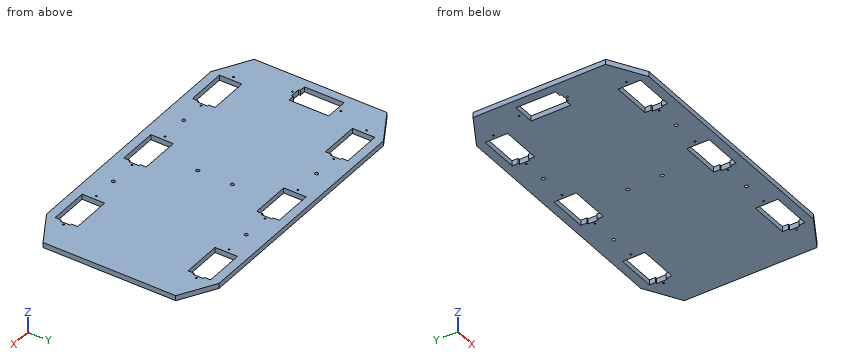
```python
from build123d import *

# Parameters (mm, degrees)
BOSS_EXTRUDE1_DEPTH = 3
CUT_EXTRUDE1_REACH  = 105
SKETCH2_R           = 0.5
SKETCH2_R_2         = 1
CUT_EXTRUDE2_REACH  = 105
SKETCH3_R           = 0.5
CUT_EXTRUDE3_REACH  = 105
SKETCH5_R           = 1


with BuildPart() as part:
    # Sketch1 → Boss-Extrude1 (new body)
    with BuildSketch(Plane.XY):
        Polygon((70, 50), (90, 38.452994616), (90, -38.452994616), (70, -50), (-70, -50), (-90, -38.452994616), (-90, 38.452994616), (-70, 50), align=None)
    extrude(amount=BOSS_EXTRUDE1_DEPTH)

    # Sketch2 → Cut-Extrude1 (cut, up to next)
    with BuildSketch(Plane.XY.offset(3), mode=Mode.PRIVATE) as cut_extrude1_sk1:
        with Locations((-72.5, 38.5)):
            Circle(SKETCH2_R)
    cut_extrude1_tool1 = extrude(cut_extrude1_sk1.sketch, amount=-CUT_EXTRUDE1_REACH, mode=Mode.PRIVATE) & part.part
    # Sketch2 → Cut-Extrude1 (cut, up to next)
    with BuildSketch(Plane.XY.offset(3), mode=Mode.PRIVATE) as cut_extrude1_sk2:
        with Locations((-44.5, 38.5)):
            Circle(SKETCH2_R)
    cut_extrude1_tool2 = extrude(cut_extrude1_sk2.sketch, amount=-CUT_EXTRUDE1_REACH, mode=Mode.PRIVATE) & part.part
    # Sketch2 → Cut-Extrude1 (cut, up to next)
    with BuildSketch(Plane.XY.offset(3), mode=Mode.PRIVATE) as cut_extrude1_sk3:
        with Locations((-14, 38.5)):
            Circle(SKETCH2_R)
    cut_extrude1_tool3 = extrude(cut_extrude1_sk3.sketch, amount=-CUT_EXTRUDE1_REACH, mode=Mode.PRIVATE) & part.part
    # Sketch2 → Cut-Extrude1 (cut, up to next)
    with BuildSketch(Plane.XY.offset(3), mode=Mode.PRIVATE) as cut_extrude1_sk4:
        with Locations((14, 38.5)):
            Circle(SKETCH2_R)
    cut_extrude1_tool4 = extrude(cut_extrude1_sk4.sketch, amount=-CUT_EXTRUDE1_REACH, mode=Mode.PRIVATE) & part.part
    # Sketch2 → Cut-Extrude1 (cut, up to next)
    with BuildSketch(Plane.XY.offset(3), mode=Mode.PRIVATE) as cut_extrude1_sk5:
        with Locations((44.5, 38.5)):
            Circle(SKETCH2_R)
    cut_extrude1_tool5 = extrude(cut_extrude1_sk5.sketch, amount=-CUT_EXTRUDE1_REACH, mode=Mode.PRIVATE) & part.part
    # Sketch2 → Cut-Extrude1 (cut, up to next)
    with BuildSketch(Plane.XY.offset(3), mode=Mode.PRIVATE) as cut_extrude1_sk6:
        with Locations((72.5, 38.5)):
            Circle(SKETCH2_R)
    cut_extrude1_tool6 = extrude(cut_extrude1_sk6.sketch, amount=-CUT_EXTRUDE1_REACH, mode=Mode.PRIVATE) & part.part
    # Sketch2 → Cut-Extrude1 (cut, up to next)
    with BuildSketch(Plane.XY.offset(3), mode=Mode.PRIVATE) as cut_extrude1_sk7:
        with Locations((72.5, -38.5)):
            Circle(SKETCH2_R)
    cut_extrude1_tool7 = extrude(cut_extrude1_sk7.sketch, amount=-CUT_EXTRUDE1_REACH, mode=Mode.PRIVATE) & part.part
    # Sketch2 → Cut-Extrude1 (cut, up to next)
    with BuildSketch(Plane.XY.offset(3), mode=Mode.PRIVATE) as cut_extrude1_sk8:
        with Locations((44.5, -38.5)):
            Circle(SKETCH2_R)
    cut_extrude1_tool8 = extrude(cut_extrude1_sk8.sketch, amount=-CUT_EXTRUDE1_REACH, mode=Mode.PRIVATE) & part.part
    # Sketch2 → Cut-Extrude1 (cut, up to next)
    with BuildSketch(Plane.XY.offset(3), mode=Mode.PRIVATE) as cut_extrude1_sk9:
        with Locations((14, -38.5)):
            Circle(SKETCH2_R)
    cut_extrude1_tool9 = extrude(cut_extrude1_sk9.sketch, amount=-CUT_EXTRUDE1_REACH, mode=Mode.PRIVATE) & part.part
    # Sketch2 → Cut-Extrude1 (cut, up to next)
    with BuildSketch(Plane.XY.offset(3), mode=Mode.PRIVATE) as cut_extrude1_sk10:
        with Locations((-14, -38.5)):
            Circle(SKETCH2_R)
    cut_extrude1_tool10 = extrude(cut_extrude1_sk10.sketch, amount=-CUT_EXTRUDE1_REACH, mode=Mode.PRIVATE) & part.part
    # Sketch2 → Cut-Extrude1 (cut, up to next)
    with BuildSketch(Plane.XY.offset(3), mode=Mode.PRIVATE) as cut_extrude1_sk11:
        with Locations((-44.5, -38.5)):
            Circle(SKETCH2_R)
    cut_extrude1_tool11 = extrude(cut_extrude1_sk11.sketch, amount=-CUT_EXTRUDE1_REACH, mode=Mode.PRIVATE) & part.part
    # Sketch2 → Cut-Extrude1 (cut, up to next)
    with BuildSketch(Plane.XY.offset(3), mode=Mode.PRIVATE) as cut_extrude1_sk12:
        with Locations((-72.5, -38.5)):
            Circle(SKETCH2_R)
    cut_extrude1_tool12 = extrude(cut_extrude1_sk12.sketch, amount=-CUT_EXTRUDE1_REACH, mode=Mode.PRIVATE) & part.part
    # Sketch2 → Cut-Extrude1 (cut, up to next)
    with BuildSketch(Plane.XY.offset(3), mode=Mode.PRIVATE) as cut_extrude1_sk13:
        with Locations((0, 10)):
            Circle(SKETCH2_R_2)
    cut_extrude1_tool13 = extrude(cut_extrude1_sk13.sketch, amount=-CUT_EXTRUDE1_REACH, mode=Mode.PRIVATE) & part.part
    # Sketch2 → Cut-Extrude1 (cut, up to next)
    with BuildSketch(Plane.XY.offset(3), mode=Mode.PRIVATE) as cut_extrude1_sk14:
        with Locations((0, -10)):
            Circle(SKETCH2_R_2)
    cut_extrude1_tool14 = extrude(cut_extrude1_sk14.sketch, amount=-CUT_EXTRUDE1_REACH, mode=Mode.PRIVATE) & part.part
    # Sketch2 → Cut-Extrude1 (cut, up to next)
    with BuildSketch(Plane.XY.offset(3), mode=Mode.PRIVATE) as cut_extrude1_sk15:
        Polygon((-11.5, 45), (11.5, 45), (11.5, 41.5), (12.5, 41.5), (12.5, 35.5), (11.5, 35.5), (11.5, 32), (-11.5, 32), align=None)
    cut_extrude1_tool15 = extrude(cut_extrude1_sk15.sketch, amount=-CUT_EXTRUDE1_REACH, mode=Mode.PRIVATE) & part.part
    # Sketch2 → Cut-Extrude1 (cut, up to next)
    with BuildSketch(Plane.XY.offset(3), mode=Mode.PRIVATE) as cut_extrude1_sk16:
        Polygon((-11.5, -32), (11.5, -32), (11.5, -35.5), (12.5, -35.5), (12.5, -41.5), (11.5, -41.5), (11.5, -45), (-11.5, -45), align=None)
    cut_extrude1_tool16 = extrude(cut_extrude1_sk16.sketch, amount=-CUT_EXTRUDE1_REACH, mode=Mode.PRIVATE) & part.part
    # Sketch2 → Cut-Extrude1 (cut, up to next)
    with BuildSketch(Plane.XY.offset(3), mode=Mode.PRIVATE) as cut_extrude1_sk17:
        Polygon((-70, 45), (-47, 45), (-47, 41.5), (-46, 41.5), (-46, 35.5), (-47, 35.5), (-47, 32), (-70, 32), align=None)
    cut_extrude1_tool17 = extrude(cut_extrude1_sk17.sketch, amount=-CUT_EXTRUDE1_REACH, mode=Mode.PRIVATE) & part.part
    # Sketch2 → Cut-Extrude1 (cut, up to next)
    with BuildSketch(Plane.XY.offset(3), mode=Mode.PRIVATE) as cut_extrude1_sk18:
        Polygon((-70, -32), (-47, -32), (-47, -35.5), (-46, -35.5), (-46, -41.5), (-47, -41.5), (-47, -45), (-70, -45), align=None)
    cut_extrude1_tool18 = extrude(cut_extrude1_sk18.sketch, amount=-CUT_EXTRUDE1_REACH, mode=Mode.PRIVATE) & part.part
    # Sketch2 → Cut-Extrude1 (cut, up to next)
    with BuildSketch(Plane.XY.offset(3), mode=Mode.PRIVATE) as cut_extrude1_sk19:
        Polygon((70, -32), (47, -32), (47, -45), (70, -45), (70, -41.5), (71, -41.5), (71, -35.5), (70, -35.5), align=None)
    cut_extrude1_tool19 = extrude(cut_extrude1_sk19.sketch, amount=-CUT_EXTRUDE1_REACH, mode=Mode.PRIVATE) & part.part
    # Sketch2 → Cut-Extrude1 (cut, up to next)
    with BuildSketch(Plane.XY.offset(3), mode=Mode.PRIVATE) as cut_extrude1_sk20:
        Polygon((70, 45), (47, 45), (47, 32), (70, 32), (70, 35.5), (71, 35.5), (71, 41.5), (70, 41.5), align=None)
    cut_extrude1_tool20 = extrude(cut_extrude1_sk20.sketch, amount=-CUT_EXTRUDE1_REACH, mode=Mode.PRIVATE) & part.part
    add(cut_extrude1_tool1.solids().sort_by_distance((-72.5, 38.5, 3))[0], mode=Mode.SUBTRACT)
    add(cut_extrude1_tool2.solids().sort_by_distance((-44.5, 38.5, 3))[0], mode=Mode.SUBTRACT)
    add(cut_extrude1_tool3.solids().sort_by_distance((-14, 38.5, 3))[0], mode=Mode.SUBTRACT)
    add(cut_extrude1_tool4.solids().sort_by_distance((14, 38.5, 3))[0], mode=Mode.SUBTRACT)
    add(cut_extrude1_tool5.solids().sort_by_distance((44.5, 38.5, 3))[0], mode=Mode.SUBTRACT)
    add(cut_extrude1_tool6.solids().sort_by_distance((72.5, 38.5, 3))[0], mode=Mode.SUBTRACT)
    add(cut_extrude1_tool7.solids().sort_by_distance((72.5, -38.5, 3))[0], mode=Mode.SUBTRACT)
    add(cut_extrude1_tool8.solids().sort_by_distance((44.5, -38.5, 3))[0], mode=Mode.SUBTRACT)
    add(cut_extrude1_tool9.solids().sort_by_distance((14, -38.5, 3))[0], mode=Mode.SUBTRACT)
    add(cut_extrude1_tool10.solids().sort_by_distance((-14, -38.5, 3))[0], mode=Mode.SUBTRACT)
    add(cut_extrude1_tool11.solids().sort_by_distance((-44.5, -38.5, 3))[0], mode=Mode.SUBTRACT)
    add(cut_extrude1_tool12.solids().sort_by_distance((-72.5, -38.5, 3))[0], mode=Mode.SUBTRACT)
    add(cut_extrude1_tool13.solids().sort_by_distance((0, 10, 3))[0], mode=Mode.SUBTRACT)
    add(cut_extrude1_tool14.solids().sort_by_distance((0, -10, 3))[0], mode=Mode.SUBTRACT)
    add(cut_extrude1_tool15.solids().sort_by_distance((0.236066, 38.5, 3))[0], mode=Mode.SUBTRACT)
    add(cut_extrude1_tool16.solids().sort_by_distance((0.236066, -38.5, 3))[0], mode=Mode.SUBTRACT)
    add(cut_extrude1_tool17.solids().sort_by_distance((-58.263934, 38.5, 3))[0], mode=Mode.SUBTRACT)
    add(cut_extrude1_tool18.solids().sort_by_distance((-58.263934, -38.5, 3))[0], mode=Mode.SUBTRACT)
    add(cut_extrude1_tool19.solids().sort_by_distance((58.736066, -38.5, 3))[0], mode=Mode.SUBTRACT)
    add(cut_extrude1_tool20.solids().sort_by_distance((58.736066, 38.5, 3))[0], mode=Mode.SUBTRACT)

    # Sketch3 → Cut-Extrude2 (cut, up to next)
    with BuildSketch(Plane.XY.offset(3), mode=Mode.PRIVATE) as cut_extrude2_sk1:
        with Locations((-78.5, 19.5)):
            Circle(SKETCH3_R)
    cut_extrude2_tool1 = extrude(cut_extrude2_sk1.sketch, amount=-CUT_EXTRUDE2_REACH, mode=Mode.PRIVATE) & part.part
    # Sketch3 → Cut-Extrude2 (cut, up to next)
    with BuildSketch(Plane.XY.offset(3), mode=Mode.PRIVATE) as cut_extrude2_sk2:
        with Locations((-78.5, -8.5)):
            Circle(SKETCH3_R)
    cut_extrude2_tool2 = extrude(cut_extrude2_sk2.sketch, amount=-CUT_EXTRUDE2_REACH, mode=Mode.PRIVATE) & part.part
    # Sketch3 → Cut-Extrude2 (cut, up to next)
    with BuildSketch(Plane.XY.offset(3), mode=Mode.PRIVATE) as cut_extrude2_sk3:
        Polygon((-85, 17), (-72, 17), (-72, -6), (-75.5, -6), (-75.5, -7), (-81.5, -7), (-81.5, -6), (-85, -6), align=None)
    cut_extrude2_tool3 = extrude(cut_extrude2_sk3.sketch, amount=-CUT_EXTRUDE2_REACH, mode=Mode.PRIVATE) & part.part
    add(cut_extrude2_tool1.solids().sort_by_distance((-78.5, 19.5, 3))[0], mode=Mode.SUBTRACT)
    add(cut_extrude2_tool2.solids().sort_by_distance((-78.5, -8.5, 3))[0], mode=Mode.SUBTRACT)
    add(cut_extrude2_tool3.solids().sort_by_distance((-78.5, 5.263934, 3))[0], mode=Mode.SUBTRACT)

    # Sketch5 → Cut-Extrude3 (cut, up to next)
    with BuildSketch(Plane(origin=(0, 0, 0), x_dir=(-1, 0, 0), z_dir=(0, 0, -1)), mode=Mode.PRIVATE) as cut_extrude3_sk1:
        with Locations((30, 38.5)):
            Circle(SKETCH5_R)
    cut_extrude3_tool1 = extrude(cut_extrude3_sk1.sketch, amount=-CUT_EXTRUDE3_REACH, mode=Mode.PRIVATE) & part.part
    # Sketch5 → Cut-Extrude3 (cut, up to next)
    with BuildSketch(Plane(origin=(0, 0, 0), x_dir=(-1, 0, 0), z_dir=(0, 0, -1)), mode=Mode.PRIVATE) as cut_extrude3_sk2:
        with Locations((-30, 38.5)):
            Circle(SKETCH5_R)
    cut_extrude3_tool2 = extrude(cut_extrude3_sk2.sketch, amount=-CUT_EXTRUDE3_REACH, mode=Mode.PRIVATE) & part.part
    # Sketch5 → Cut-Extrude3 (cut, up to next)
    with BuildSketch(Plane(origin=(0, 0, 0), x_dir=(-1, 0, 0), z_dir=(0, 0, -1)), mode=Mode.PRIVATE) as cut_extrude3_sk3:
        with Locations((30, -38.5)):
            Circle(SKETCH5_R)
    cut_extrude3_tool3 = extrude(cut_extrude3_sk3.sketch, amount=-CUT_EXTRUDE3_REACH, mode=Mode.PRIVATE) & part.part
    # Sketch5 → Cut-Extrude3 (cut, up to next)
    with BuildSketch(Plane(origin=(0, 0, 0), x_dir=(-1, 0, 0), z_dir=(0, 0, -1)), mode=Mode.PRIVATE) as cut_extrude3_sk4:
        with Locations((-30, -38.5)):
            Circle(SKETCH5_R)
    cut_extrude3_tool4 = extrude(cut_extrude3_sk4.sketch, amount=-CUT_EXTRUDE3_REACH, mode=Mode.PRIVATE) & part.part
    add(cut_extrude3_tool1.solids().sort_by_distance((-30, 38.5, 0))[0], mode=Mode.SUBTRACT)
    add(cut_extrude3_tool2.solids().sort_by_distance((30, 38.5, 0))[0], mode=Mode.SUBTRACT)
    add(cut_extrude3_tool3.solids().sort_by_distance((-30, -38.5, 0))[0], mode=Mode.SUBTRACT)
    add(cut_extrude3_tool4.solids().sort_by_distance((30, -38.5, 0))[0], mode=Mode.SUBTRACT)


solid = part.part
```
Check sheet for the modelled part. Datum: model origin and axes. Units: mm. Coordinates: 2 decimals unless noted, no trailing zeros. Order: outer loops, then holes, each group sorted by start corner. A loop starts at its lowest first (then second) coordinate and runs counter-clockwise, first axis right, second up. Notation, with made-up numbers: (70.5, -25) -> (80.5, -25) arc R18 ccw to (80.5, -3) -> close; hole circle Ø3 at (84, -1). An arc over 180 degrees is marked (long way). Write item = value, one per line. Start each with the question number.
1) Cross-section at A-A (x = 56.5). Enter the section's corners in (y, z), then the cut area to 3 significant figures.
2) Cross-section at B-B (y = 0). Enter the section's corners in (x, z), then the cut area to 3 significant figures.
3) Go/stop test with flat-tipped pins: P1, Ø0.9, axis at y = 43.5, z = 1, coming from the -X side; P2, Ø1.5, axis at y = 39.5, z = 1, coming from the +X side. Record where each tip stops, or that it passes through.
4) Material ranges on L1, parallel to Y at x = -14, z = 1.3; L2, parallel to Y at x = -56, z = 1.8; L3, parallel to X at y = 35, z = 0.4, recorded low to high.
5) Cross-section at C-C (z = 2). State how many separate pieces and enclosed holes the cut face has, then the cut area to 3 significant figures.
Ans:
q1.outline = (-50, 0) -> (-45, 0) -> (-45, 3) -> (-50, 3) -> close; (-32, 0) -> (32, 0) -> (32, 3) -> (-32, 3) -> close; (45, 0) -> (50, 0) -> (50, 3) -> (45, 3) -> close
q1.area = 222 mm²
q2.outline = (-90, 0) -> (-85, 0) -> (-85, 3) -> (-90, 3) -> close; (-72, 0) -> (90, 0) -> (90, 3) -> (-72, 3) -> close
q2.area = 501 mm²
q3.P1 = -82.04
q3.P2 = 89.49
q4.L1 = -50 to -39, -38 to 38, 39 to 50
q4.L2 = -50 to -45, -32 to 32, 45 to 50
q4.L3 = -90 to -70, -47 to -11.5, 11.5 to 47, 70 to 90
q5.separate_pieces = 1
q5.enclosed_holes = 27
q5.area = 15,400 mm²
